```python
from build123d import *

# Parameters (mm, degrees)
PAD_DEPTH       = 8.3
SKETCH001_R     = 0.9
POCKET_DEPTH    = 10
PAD001_DEPTH    = 5
SKETCH003_W     = 8.001678
SKETCH003_H     = 6.862923
POCKET001_DEPTH = 5


with BuildPart() as part:
    # Sketch → Pad (new body)
    with BuildSketch(Plane.XY):
        with BuildLine():
            Line((-84.1375, 3.25), (72, 3.25))
            Line((72, 3.25), (72, 6.94))
            ThreePointArc((74.47, 6.940013), (73.234993, 8.174999), (72, 6.94))
            Line((74.47, 6.940013), (74.47, 3.250013))
            Line((74.47, 3.250013), (84.1375, 3.25))
            Line((84.1375, 3.25), (84.1375, -3.25))
            Line((84.1375, -3.25), (-72, -3.25))
            Line((-72, -3.25), (-72, -6.94))
            ThreePointArc((-74.47, -6.94), (-73.235, -8.175005), (-72, -6.94))
            Line((-74.47, -6.94), (-74.47, -3.25))
            Line((-74.47, -3.25), (-84.1375, -3.25))
            Line((-84.1375, -3.25), (-84.1375, 3.25))
        make_face()
    extrude(amount=PAD_DEPTH)

    # Sketch001 (on Face14 of Pad) → Pocket (cut)
    with BuildSketch(Plane.XY.offset(8.3)):
        with Locations((-81.61, 0)):
            Circle(SKETCH001_R)
        with Locations((-79.07, 0)):
            Circle(SKETCH001_R)
        with Locations((-66.993, 0)):
            Circle(SKETCH001_R)
        with Locations((-64.453, 0)):
            Circle(SKETCH001_R)
        with Locations((-52.376, 0)):
            Circle(SKETCH001_R)
        with Locations((-49.836, 0)):
            Circle(SKETCH001_R)
        with Locations((-37.759, 0)):
            Circle(SKETCH001_R)
        with Locations((-35.219, 0)):
            Circle(SKETCH001_R)
        with Locations((-23.142, 0)):
            Circle(SKETCH001_R)
        with Locations((-20.602, 0)):
            Circle(SKETCH001_R)
        with Locations((-8.525, 0)):
            Circle(SKETCH001_R)
        with Locations((-5.985, 0)):
            Circle(SKETCH001_R)
        with Locations((6.092, 0)):
            Circle(SKETCH001_R)
        with Locations((8.632, 0)):
            Circle(SKETCH001_R)
        with Locations((20.709, 0)):
            Circle(SKETCH001_R)
        with Locations((23.249, 0)):
            Circle(SKETCH001_R)
        with Locations((35.326, 0)):
            Circle(SKETCH001_R)
        with Locations((37.866, 0)):
            Circle(SKETCH001_R)
        with Locations((49.943, 0)):
            Circle(SKETCH001_R)
        with Locations((52.483, 0)):
            Circle(SKETCH001_R)
        with Locations((64.56, 0)):
            Circle(SKETCH001_R)
        with Locations((67.1, 0)):
            Circle(SKETCH001_R)
        with Locations((79.177, 0)):
            Circle(SKETCH001_R)
        with Locations((81.717, 0)):
            Circle(SKETCH001_R)
    extrude(amount=-POCKET_DEPTH, mode=Mode.SUBTRACT)

    # Sketch002 (on Face5 of Pocket) → Pad001 (join)
    with BuildSketch(Plane.XY.offset(8.3)):
        with BuildLine():
            Line((74.47, 6.97), (74.47, 5.7))
            ThreePointArc((72, 5.7), (73.235, 4.465), (74.47, 5.7))
            Line((72, 5.7), (72, 6.97))
            ThreePointArc((74.47, 6.97), (73.235, 8.204992), (72, 6.97))
        make_face()
        with BuildLine():
            Line((-72, -5.7), (-72, -6.97))
            ThreePointArc((-74.47, -6.97), (-73.235, -8.205), (-72, -6.97))
            Line((-74.47, -6.97), (-74.47, -5.7))
            ThreePointArc((-72, -5.7), (-73.235, -4.465), (-74.47, -5.7))
        make_face()
    extrude(amount=PAD001_DEPTH)

    # Sketch003 (on Face4 of Pad001) → Pocket001 (cut)
    with BuildSketch(Plane(origin=(0, 0, 0), x_dir=(1, 0, 0), z_dir=(0, 0, -1))):
        with Locations((73.336792, -6.681462)):
            Rectangle(SKETCH003_W, SKETCH003_H)
    extrude(amount=-POCKET001_DEPTH, mode=Mode.SUBTRACT)


solid = part.part
```
Here's how the part is built. I have some questions about the finished solid (model axes, mm). A direction names the side the tool comes from. Give positions to 0.01 mm unless a question says otherwise; leave off trailing zeros. Loops run counter-clockwise (first coordinate to the right, second up) from the corner with the lowest first, then second, coordinate; pieces in that order, holes last. Notation, with made-up numbers: (14, 40) -> (20, 40) arc R28 ccw to (20, 61) -> close; hole circle Ø2 at (60.25, 72.5). An arc over 180 degrees is marked (long way). Use one line per item in the form item = value. Start each with the question number.
1) Imagine slicing it at A-A (z = 9.75). Please give me the cut outline in (x, y) (3 decimals).
2) Thinking about a two-plate mould opening in Z: for faces 1 (the face through (1, 0, 8.3)), 2 (the face through (73, 6, 5)), 3 (the face through (-7, 3.25, 4)), which applies, +Z half, -Z half, draft (parallel to the pull), parting line (faces both ways), or undercut?
3) For P1, Ø6, axis at x = 43, z = 7.5, coming from the -Y side; P2, Ø6.5, axis at x = 21.5, z = 6, coming from the +Y side; P3, Ø1.4, axis at x = -49.836, y = 0, coming from the -Z side; P4, Ø8, axis at x = -28, y = -2.5, coming from the +Z side, each with a flat end and sliding along its axis, tell me the tip position at first contact or that it passes through.
4) Which directions (+Z, -Z, +X, -X, +Y, -Y) give clear straight access to the entire face, cutting with the end or side of a thin tool? Please do faces 4 (the face through (74.47, 6, 8)), 5 (the face through (7, -3.25, 4)), 6 (the face through (-74.47, -5, 5)).
5) Imagine slicing it at B-B (z = 3). Count the separate pieces of the cut face and the enclosed holes in it, then the cut area to 3 significant figures.
6) Please list where these lines run through material, in increasing order: line 1 along Y through (x, z) = (38, 4.75); line 2 along Z through (x, y) = (-6, 2); line 3 along X through (y, z) = (-6.75, 6).
Check values:
q1.outline = (-74.47, -6.97) arc R1.235 ccw to (-72, -6.97) -> (-72, -5.7) arc R1.235 ccw to (-74.47, -5.7) -> close; (72, 5.7) arc R1.235 ccw to (74.47, 5.7) -> (74.47, 6.97) arc R1.235 ccw to (72, 6.97) -> close
q2.face_1 = +Z half
q2.face_2 = -Z half
q2.face_3 = draft
q3.P1 = -3.25
q3.P2 = 3.25
q3.P3 = through
q3.P4 = 8.3
q4.face_4 = +Z, -Z, +X, +Y
q4.face_5 = +Z, -Z, +X, -Y
q4.face_6 = +Z, -Z, -X, -Y
q5.separate_pieces = 1
q5.enclosed_holes = 24
q5.area = 1,040 mm^2
q6.line_1 = -3.25 to -0.89, 0.89 to 3.25
q6.line_2 = 0 to 8.3
q6.line_3 = -74.47 to -72
